```python
from build123d import *

# Parameters (mm, degrees)
BOSS_EXTRUDE1_DEPTH       = 10.9
M3X0_5_TAPPED_HOLE1_D     = 2.5
M3X0_5_TAPPED_HOLE1_DEPTH = 20
M3X0_5_TAPPED_HOLE1_TIP   = 0.751075774


with BuildPart() as part:
    # Sketch1 → Boss-Extrude1 (new body)
    with BuildSketch(Plane(origin=(0, 0, 0), x_dir=(1, 0, 0), z_dir=(0, 1, 0))):
        Polygon((3.226233304, 0), (1.613116652, 2.794), (-1.613116652, 2.794), (-3.226233304, 0), (-1.613116652, -2.794), (1.613116652, -2.794), align=None)
    extrude(amount=BOSS_EXTRUDE1_DEPTH)

    # M3x0.5 Tapped Hole1
    with Locations(Plane(origin=(0, 10.9, 0), x_dir=(1, 0, 0), z_dir=(0, 1, 0))):
        with Locations((0, 0)):
            Hole(M3X0_5_TAPPED_HOLE1_D / 2, depth=M3X0_5_TAPPED_HOLE1_DEPTH)
            with Locations((0, 0, -(M3X0_5_TAPPED_HOLE1_DEPTH + M3X0_5_TAPPED_HOLE1_TIP / 2))):  # 118° drill point
                Cone(0, M3X0_5_TAPPED_HOLE1_D / 2, M3X0_5_TAPPED_HOLE1_TIP, mode=Mode.SUBTRACT)


solid = part.part
```
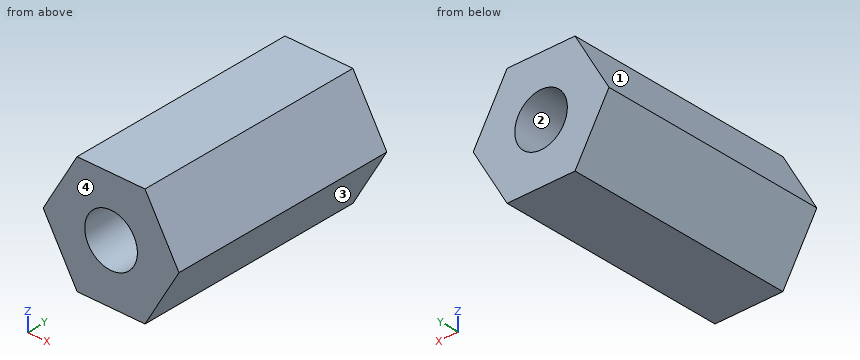
Design review of the part built by this model. Coordinates are the model's own, in mm. Face numbers are marked on the shaded views. Coordinates: 2 decimals unless noted, no trailing zeros. Order: outer loops, then holes, each group sorted by start corner. A loop starts at its lowest first (then second) coordinate and runs counter-clockwise, first axis right, second up. Notation, with made-up numbers: M -6,-9 L 25,-9 A30 cw 25,27 Z; hole C 29.5,24.25 d6. An arc over 180 degrees is marked long. Answer as a JSON object with one key per item and string values. Group by question number.
1) Add section D-D, the plane x = 2.5. Write out the cut boundary in (y, z), then the cut area to 3 significant figures.
2) Wall thickness on L1, parallel to Z at x = 0, y = 8; L2, parallel to Z at x = 0.75, y = 5.75; L3, parallel to X at y = 10, z = 0.05: over which ranges is each line inside the solid? List them lowest first.
3) Add section C-C, the plane z = -1.6. Write out the cut boundary in (x, y).
4) Mouldability with a two-part tool opening along X and no side actions: class the marked faces 1, 2, 3 and 4 as pulls with the +X half, pulls with the -X half, needs draft (parallel to the pull), parting line crosses it, or undercut.
5) Add section A-A, the plane x = -0.25. Write out the cut boundary in (y, z).
6) Add section B-B, the plane z = 0.2. Write out the cut boundary in (x, y).
Computed values:
{
 "1": {"outline": "M 0,-1.26 L 10.9,-1.26 L 10.9,1.26 L 0,1.26 Z", "area": "27.4 mm^2"},
 "2": {"L1": "z = -2.79 to -1.25, 1.25 to 2.79", "L2": "z = -2.79 to -1, 1 to 2.79", "L3": "x = -3.2 to -1.25, 1.25 to 3.2"},
 "3": {"outline": "M -2.3,0 L 2.3,0 L 2.3,10.9 L -2.3,10.9 Z"},
 "4": {"face 1": "pulls with the -X half", "face 2": "undercut", "face 3": "pulls with the +X half", "face 4": "needs draft"},
 "5": {"outline": "M 0,-2.79 L 10.9,-2.79 L 10.9,-1.22 L 0,-1.22 Z; M 0,1.22 L 10.9,1.22 L 10.9,2.79 L 0,2.79 Z"},
 "6": {"outline": "M -3.11,0 L -1.23,0 L -1.23,10.9 L -3.11,10.9 Z; M 1.23,0 L 3.11,0 L 3.11,10.9 L 1.23,10.9 Z"}
}
